from build123d import *

# Parameters (mm, degrees)
F7_DEPTH  = 12
F3_W      = 18.5
F3_H      = 9
F5_R      = 1
F2_W      = 30
F2_H      = 9
F0_W      = 51
F0_H      = 1
F8_DEPTH  = 12
F9_DEPTH  = 9
F10_DEPTH = 3
F11_R     = 2.99999
F13_R     = 2
F12_R     = 2
F14_DEPTH = 23.9
F15_SIZE  = 2
F1_W      = 13
F1_H      = 13
F16_DEPTH = 10


# Not quite as in the source:
# - a fillet or chamfer is up to 0.001 mm smaller than in the source, because OpenCascade refuses the exact size


with BuildPart() as f7:
    # F6 (on Top) → F7 (new body)
    with BuildSketch(Plane.XY):
        Polygon((58.3547055721, 23.1172949925), (-78.9411039278, 23.1172949925), (-78.9411039278, 21.0728161037), (-66.9411039278, 21.0728161037), (-66.9411039278, 5.1172949925), (-64.9411039278, 5.1172949925), (-64.9411039278, 9.1172949925), (-51.9411039278, 9.1172949925), (-45.9411039278, 9.0077459167), (-26.9411039278, 9.0077459167), (-26.9411039278, 5.1172949925), (55.6804920286, 5.1172949925), (55.6804920286, 21.0728161037), (67.6804920286, 21.0728161037), (67.6804920286, 23.1172949925), align=None)
    extrude(amount=F7_DEPTH)

    # F4 (on Top) + F3 (on Top) + F5 (on Top) + F2 (on Top) + F0 (on Top) → F8 (cut)
    with BuildSketch(Plane.XY):
        Polygon((-22.3430277164, 7.1172949925), (-21.4770023127, 8.6172949925), (-22.3430277164, 10.1172949925), (-24.075078524, 10.1172949925), (-24.9411039278, 8.6172949925), (-24.075078524, 7.1172949925), align=None)
    with BuildSketch(Plane.XY):
        with Locations((-23.5695079714, 16.6172949925)):
            Rectangle(F3_W, F3_H)
    with BuildSketch(Plane.XY):
        with Locations((-17.0899687546, 9.1172949925)):
            Circle(F5_R)
    with BuildSketch(Plane.XY):
        with Locations((-49.9411039278, 16.6172949925)):
            Rectangle(F2_W, F2_H)
    with BuildSketch(Plane.XY):
        with Locations((28.1804920286, 8.6172949925)):
            Rectangle(F0_W, F0_H)
    extrude(amount=F8_DEPTH, mode=Mode.SUBTRACT)

    # F6 (on Top) → F9 (join)
    with BuildSketch(Plane.XY):
        Polygon((-51.9411039278, 9.1172949925), (-51.9411039278, 5.1172949925), (-45.9411039278, 5.1172949925), (-45.9411039278, 9.0077459167), align=None)
    extrude(amount=F9_DEPTH)

    # F6 (on Top) → F10 (cut)
    with BuildSketch(Plane.XY):
        Polygon((-51.9411039278, 9.1172949925), (-51.9411039278, 5.1172949925), (-45.9411039278, 5.1172949925), (-45.9411039278, 9.0077459167), align=None)
    extrude(amount=F10_DEPTH, mode=Mode.SUBTRACT)

    # F11 (radius 3 in the source; OpenCascade refuses exactly that, so slightly less here)
    f11_edges = [f7.edges().sort_by_distance(p)[0] for p in [
        (-51.941104, 7.117295, 9),
        (-45.941104, 7.06252, 9),
        (-51.941104, 7.117295, 3),
        (-45.941104, 7.06252, 3),
    ]]
    fillet(f11_edges, radius=F11_R)

    # F13 (on Front) + F12 (on Front) → F14 (cut)
    with BuildSketch(Plane.XZ):
        with Locations((-72.9411039278, 6)):
            Circle(F13_R)
    with BuildSketch(Plane.XZ):
        with Locations((61.6804920286, 6)):
            Circle(F12_R)
    extrude(amount=-F14_DEPTH, mode=Mode.SUBTRACT)

    # F15
    f15_edges = [f7.edges().sort_by_distance(p)[0] for p in [
        (-74.941104, 21.072816, 6),
        (59.680492, 21.072816, 6),
    ]]
    chamfer(f15_edges, length=F15_SIZE)

    # F1 (on Top) → F16 (cut)
    with BuildSketch(Plane.XY):
        with Locations((-5.8195079714, 14.6172949925)):
            Rectangle(F1_W, F1_H)
    extrude(amount=F16_DEPTH, mode=Mode.SUBTRACT)


solid = f7.part
Here's how the part is built. I have some questions about the finished solid (model axes, mm). A direction names the side the tool comes from. Give positions to 0.01 mm unless a question says otherwise; leave off trailing zeros. Order: outer loops, then holes, each group sorted by start corner. A loop starts at its lowest first (then second) coordinate and runs counter-clockwise, first axis right, second up. Notation, with made-up numbers: (64.5, -26) -> (103.5, -26) arc R17 cw to (103.5, 7) -> close; hole circle Ø3 at (32, 20). An arc over 180 degrees is marked (long way). One line per item, written item: value. Start each with the question number.
1. Imagine slicing it at A-A, the plane y = 16.25. List the corners of the cut face in (x, z) for me, plus the area to 3 significant figures.
2. Will these pins go through, and if not, where does the flat tip stop? pin 1 Ø3.5 at (x, z) = (-40.5, 5) entering from -Y; pin 2 Ø4.5 at (y, z) = (7.5, 6.5) entering from +X; pin 3 Ø6 at (y, z) = (9, 4) entering from -X.
3. For faces 1 (the face through (57.6, 21.073, 4.6)), 2 (the face through (-46.8, 7.1, 3.9)), 3 (the face through (-24, 12.117, 6)), 4 (the face through (-26.941, 7, 6)), 5 (the face through (-74.4, 21.073, 1.9)), which set-ups out of +Z, -Z, +X, -X, +Y, -Y let a thin tool reach every point of the face, with its end or its side?
4. I need wall thicknesses on probe 1 along X at (y, z) = (20.5, 7); probe 2 along X at (y, z) = (19, 11); probe 3 along Y at (x, z) = (-44.5, 6.5). Which ranges of each line are inside material? Lowest first, please. Write a range as from..to.
5. Imagine slicing it at B-B, the plane x = 27.5. List the corners of the cut face in (y, z) for me, plus the area to 3 significant figures.
Values follow:
1. outline: (-66.94, 0) -> (-64.94, 0) -> (-64.94, 12) -> (-66.94, 12) -> close; (-34.94, 0) -> (-32.82, 0) -> (-32.82, 12) -> (-34.94, 12) -> close; (-14.32, 0) -> (-12.32, 0) -> (-12.32, 10) -> (0.68, 10) -> (0.68, 0) -> (55.68, 0) -> (55.68, 12) -> (-14.32, 12) -> close
1. area: 759 mm2
2. pin 1: stops at y = 9.01
2. pin 2: stops at x = 55.68
2. pin 3: stops at x = -66.94
3. face 1: +Z, -Z, +X, -Y
3. face 2: -Z, -Y
3. face 3: +Z, -Z
3. face 4: +Z, -Z, -Y
3. face 5: +Z, -Z, -X, -Y
4. probe 1: x = -66.94..-64.94, -34.94..-32.82, -14.32..-12.32, 0.68..55.68
4. probe 2: x = -66.94..-64.94, -34.94..-32.82, -14.32..55.68
4. probe 3: y = 9.01..12.12, 21.12..23.12
5. outline: (5.12, 0) -> (8.12, 0) -> (8.12, 12) -> (5.12, 12) -> close; (9.12, 0) -> (23.12, 0) -> (23.12, 12) -> (9.12, 12) -> close
5. area: 204 mm2
